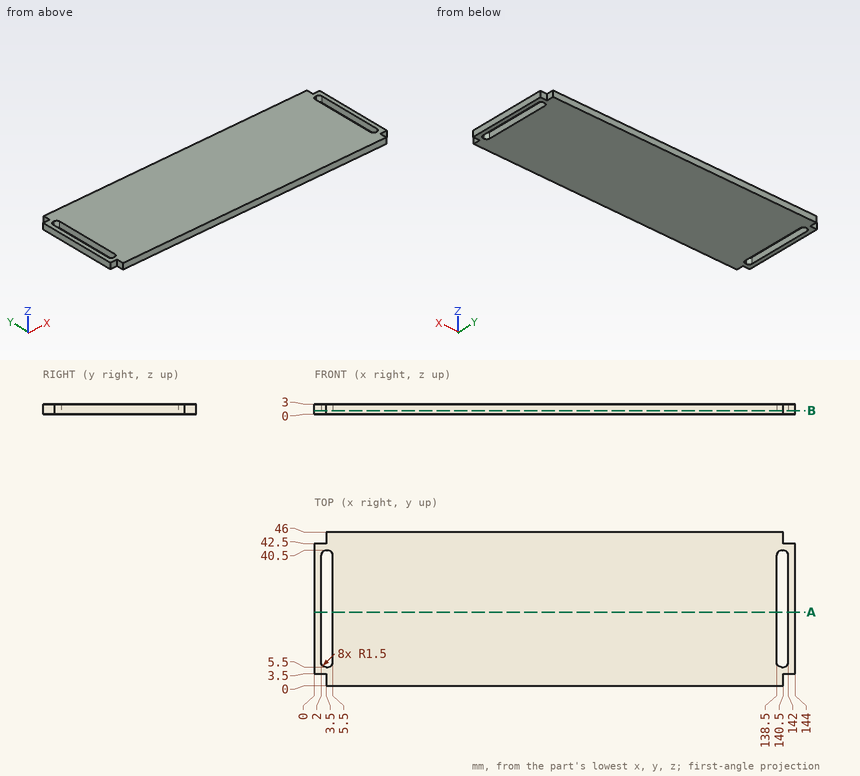
Verification items for this drawing (mm, ordinates from the low corner). Round coordinates to 2 decimals unless told otherwise and drop trailing zeros. Order: outer loops, then holes, each group sorted by start corner. A loop starts at its lowest first (then second) coordinate and runs counter-clockwise, first axis right, second up.
1) Depth check by flat-ended pin: pin 1 (1.5 mm diameter, centred on x = 143, z = 1, fed in from +Y); pin 2 (1.5 mm diameter, centred on x = 143, z = 1, fed in from -Y); pin 3 (3 mm diameter, centred on x = 40.5, y = 20.5, fed in from -Z); pin 4 (1.5 mm diameter, centred on y = 1, z = 1.5, fed in from -X). Enter the tip coordinate at first touch or a pass-through.
Geometry says:
pin 1: stops at y = 42.5
pin 2: stops at y = 3.5
pin 3: stops at z = 0
pin 4: stops at x = 3.5
2) Cross-section at B-B, the plane z = 1. Record the cut outline in (x, y).
Geometry says:
outline: (0, 3.5) - (3.5, 3.5) - (3.5, 0) - (140.5, 0) - (140.5, 3.5) - (144, 3.5) - (144, 42.5) - (140.5, 42.5) - (140.5, 46) - (3.5, 46) - (3.5, 42.5) - (0, 42.5) - close; hole (2, 7) arc R1.5 ccw to (3.5, 5.5) - (4, 5.5) arc R1.5 ccw to (5.5, 7) - (5.5, 39) arc R1.5 ccw to (4, 40.5) - (3.5, 40.5) arc R1.5 ccw to (2, 39) - close; hole (138.5, 7) arc R1.5 ccw to (140, 5.5) - (140.5, 5.5) arc R1.5 ccw to (142, 7) - (142, 39) arc R1.5 ccw to (140.5, 40.5) - (140, 40.5) arc R1.5 ccw to (138.5, 39) - close
3) Material ranges on line 1 (X direction, y = 28, z = 2.7), recorded low to high.
Geometry says:
line 1: x = 0 to 2, 5.5 to 138.5, 142 to 144
4) Cross-section at A-A, the plane y = 22. Record the cut outline in (x, z).
Geometry says:
outline: (0, 0) - (2, 0) - (2, 3) - (0, 3) - close; (5.5, 0) - (138.5, 0) - (138.5, 3) - (5.5, 3) - close; (142, 0) - (144, 0) - (144, 3) - (142, 3) - close
